Autodesk Inventor part; units mm, degrees
ref_plane "YZ Plane" through (0, 0, 0) normal (1, 0, 0) x (0, 1, 0)
ref_plane "XZ Plane" through (0, 0, 0) normal (0, 1, 0) x (-1, 0, 0)
ref_plane "XY Plane" through (0, 0, 0) normal (0, 0, 1) x (1, 0, 0)
sketch "スケッチ1" plane through (0, 0, 0) normal (0, 0, 1) x (1, 0, 0)
  circle A0 centre (0, 0) radius 1.85
  dimension "d0" = 3.7
extrude "押し出し1" add sketch "スケッチ1" along normal blind 2
sketch "スケッチ2" plane through (0, 0, 0) normal (0, 0, -1) x (-1, 0, 0)
  circle A0 centre (0, 0) radius 1
  dimension "d3" = 2
extrude "押し出し2" add sketch "スケッチ2" along normal blind 6
thread "ねじ1"
chamfer "面取り1" distance 0.3 angle 45 1 edges at (-1.85, 0, 2)
properties part number "M2×6" material "ステンレス鋼"
Work out the finished part from the listing and answer in its coordinate system (mm). A direction names the side the tool comes from. Give positions to 0.01 mm unless a question says otherwise; leave off trailing zeros. Order: outer loops, then holes, each group sorted by start corner. A loop starts at its lowest first (then second) coordinate and runs counter-clockwise, first axis right, second up. Notation, with made-up numbers: (23.5, 52.25) - (75.5, 52.25) arc R25 ccw to (75.5, 77.25) - close; hole circle Ø3 at (76, 2). An arc over 180 degrees is marked (long way). One line per item, written item: value. Start each with the question number.
1. Which of the six approach directions +Z, -Z, +X, -X, +Y, -Y give full straight-line access (tool end or side, diameter ignored) to faces 1 (the face through (0, 0, 2)), 2 (the face through (1, -1, 0))?
2. Consider line 1 (Z direction, x = 0.25, y = -1); line 2 (X direction, y = 1.6, z = 1); line 3 (X direction, y = 0.3, z = 1.25). Determine where each line is inside the solid, lowest interval first.
3. Section A-A, the plane y = 0 is taken. Write down the section's boundary in (x, z), then the cut area to 3 significant figures.
4. Section C-C, the plane z = -2.5 is taken. Write down the section's boundary in (x, y).
5. This flat-tipped pin is pushed along its axis until it touches: pin 1 Ø2 at (y, z) = (-1, -1.5) entering from -X. Where does it stop, or does it pass through?
Filled sheet:
1. face 1: +Z, +X, -X, +Y, -Y
1. face 2: -Z
2. line 1: 0 to 2
2. line 2: -0.93 to 0.93
2. line 3: -1.83 to 1.83
3. outline: (-1.85, 0) - (-1, 0) - (-1, -6) - (1, -6) - (1, 0) - (1.85, 0) - (1.85, 1.7) - (1.55, 2) - (-1.55, 2) - (-1.85, 1.7) - close
3. area: 19.3 mm²
4. outline: circle Ø2 at (0, 0)
5. pin 1: x = -1
